```python
from build123d import *

# Parameters (mm, degrees)
F1_DEPTH = 40
F2_R     = 5
F3_W     = 50
F3_H     = 40
F4_DEPTH = 1


with BuildPart() as f1:
    # F0 (on Right) → F1 (new body, symmetric)
    with BuildSketch(Plane.YZ):
        with BuildLine():
            ThreePointArc((4.6023512578, 12.0836236967), (18.5654944992, 26.0467669382), (32.5286377407, 12.0836236967))
            Line((32.5286377407, 12.0836236967), (40.2273690835, 12.0836236967))
            Line((40.2273690835, 12.0836236967), (40.2273690835, 92.0836236967))
            Line((40.2273690835, 92.0836236967), (-29.7726309165, 92.0836236967))
            Line((-29.7726309165, 92.0836236967), (-39.7726309165, 42.0836236967))
            Line((-39.7726309165, 42.0836236967), (-79.7726309165, 42.0836236967))
            Line((-79.7726309165, 42.0836236967), (-79.7726309165, 12.0836236967))
            Line((-79.7726309165, 12.0836236967), (-68.3018244008, 12.0836236967))
            ThreePointArc((-68.3018244008, 12.0836236967), (-54.4831605593, 25.9022875381), (-40.6644967179, 12.0836236967))
            Line((-40.6644967179, 12.0836236967), (4.6023512578, 12.0836236967))
        make_face()
        with BuildLine():
            Line((-68.3018244008, 12.0836236967), (-40.6644967179, 12.0836236967))
            ThreePointArc((-40.6644967179, 12.0836236967), (-54.4831605593, 25.9022875381), (-68.3018244008, 12.0836236967))
        make_face()
        with BuildLine():
            ThreePointArc((-68.3018244008, 12.0836236967), (-54.4831605593, -1.7350401447), (-40.6644967179, 12.0836236967))
            Line((-40.6644967179, 12.0836236967), (-68.3018244008, 12.0836236967))
        make_face()
        with BuildLine():
            Line((4.6023512578, 12.0836236967), (32.5286377407, 12.0836236967))
            ThreePointArc((32.5286377407, 12.0836236967), (18.5654944992, 26.0467669382), (4.6023512578, 12.0836236967))
        make_face()
        with BuildLine():
            ThreePointArc((4.6023512578, 12.0836236967), (18.5654944992, -1.8795195447), (32.5286377407, 12.0836236967))
            Line((32.5286377407, 12.0836236967), (4.6023512578, 12.0836236967))
        make_face()
    extrude(amount=F1_DEPTH, both=True)

    # F2
    f2_edges = [f1.edges().sort_by_distance(p)[0] for p in [
        (-40, -34.772631, 67.083624),
        (0, -39.772631, 42.083624),
        (40, -34.772631, 67.083624),
        (0, -29.772631, 92.083624),
        (0, -79.772631, 42.083624),
        (-40, -79.772631, 27.083624),
        (0, -79.772631, 12.083624),
        (40, -79.772631, 27.083624),
        (0, -68.301824, 12.083624),
        (-40, -54.483161, -1.73504),
        (0, -40.664497, 12.083624),
        (40, -54.483161, -1.73504),
        (-40, -59.772631, 42.083624),
        (-40, -74.037228, 12.083624),
        (-40, -18.031073, 12.083624),
        (-40, 18.565494, -1.87952),
        (-40, 36.378003, 12.083624),
        (-40, 40.227369, 52.083624),
        (-40, 5.227369, 92.083624),
        (0, 40.227369, 92.083624),
        (40, 40.227369, 52.083624),
        (0, 40.227369, 12.083624),
        (40, -59.772631, 42.083624),
        (40, -74.037228, 12.083624),
        (40, -18.031073, 12.083624),
        (40, 18.565494, -1.87952),
        (40, 36.378003, 12.083624),
        (40, 5.227369, 92.083624),
    ]]
    fillet(f2_edges, radius=F2_R)

    # F3 (on face) → F4 (cut, symmetric)
    with BuildSketch(Plane.YZ.offset(40)):
        with Locations((3.8793236017, 61.9780325047)):
            Rectangle(F3_W, F3_H)
    extrude(amount=F4_DEPTH, both=True, mode=Mode.SUBTRACT)


solid = f1.part
```
Source: CAD feature listing. Evaluate the final solid. Frame: model axes, mm. A direction names the side the tool comes from. Give positions to 0.01 mm unless a question says otherwise; leave off trailing zeros. Order: outer loops, then holes, each group sorted by start corner. A loop starts at its lowest first (then second) coordinate and runs counter-clockwise, first axis right, second up. Notation, with made-up numbers: (35.5, 82) -> (88.5, 82) arc R26 cw to (88.5, 114) -> close; hole circle Ø8 at (19, 89). An arc over 180 degrees is marked (long way). Use a Markdown table: item, result.
Q1. Pull-direction query (Y, two-part tool) for faces 1 (the face through (38.496, -12.275, 13.509)), 2 (the face through (0.49, -34.714, 67.377)), 3 (the face through (38.496, -59.538, 40.658)); classes: +Y half, -Y half, draft (parallel to the pull), parting line (faces both ways), or undercut.
A:
| item | result |
|---|---|
| face 1 | undercut |
| face 2 | -Y half |
| face 3 | draft |
Q2. First-contact query: P1, Ø5, axis at x = 28.5, y = -43, coming from the +Z side; P2, Ø0.5, axis at x = 39.5, z = 61, coming from the +Y side; P3, Ø1.1, axis at x = 39.5, y = 1.5, coming from the +Z side. Flat tips, straight axial feed; report the tip coordinate or a pass-through.
A:
| item | result |
|---|---|
| P1 | z = 43.39 |
| P2 | y = 37.86 |
| P3 | z = 90.15 |
Q3. Access query for faces 4 (the face through (0, -16, 12.084)), 5 (the face through (38.496, -73.684, 13.509)), 6 (the face through (-38.496, -59.538, 40.658)). Directions: +Z, -Z, +X, -X, +Y, -Y. A direction counts if a zero-diameter tool reaches every point of the face in a straight line with its end or side. Return the directions, or none.
A:
| item | result |
|---|---|
| face 4 | -Z, +X, -X |
| face 5 | -Z, +X, -Y |
| face 6 | +Z, -X, -Y |
Q4. Section A-A (y = -22.5). Return the cut outline in (x, z), and give its area (3 significant figures).
A:
| item | result |
|---|---|
| outline | (-40, 17.08) arc R5 ccw to (-35, 12.08) -> (35, 12.08) arc R5 ccw to (40, 17.08) -> (40, 87.08) arc R5 ccw to (35, 92.08) -> (-35, 92.08) arc R5 ccw to (-40, 87.08) -> close |
| area | 6,380 mm^2 |
Q5. Section C-C (y = -7). Return the cut outline in (x, z).
A:
| item | result |
|---|---|
| outline | (-40, 17.08) arc R5 ccw to (-35, 12.08) -> (35, 12.08) arc R5 ccw to (40, 17.08) -> (40, 41.98) -> (39, 41.98) -> (39, 81.98) -> (40, 81.98) -> (40, 87.08) arc R5 ccw to (35, 92.08) -> (-35, 92.08) arc R5 ccw to (-40, 87.08) -> close |
Q6. Material intervals for line 1 (Z direction, x = -4, y = 4.5); line 2 (Y direction, x = 35.5, z = 8.5) (3 decimals); line 3 (Y direction, x = 21, z = 3), sorted ascending. Write a range as [from, to].
A:
| item | result |
|---|---|
| line 1 | [12.08, 92.08] |
| line 2 | [-67.804, -41.162], [5.096, 32.035] |
| line 3 | [-64.9, -44.07], [7.96, 29.17] |
Q7. Section B-B (x = 22). Return the cut outline in (y, z), and give its area (3 significant figures).
A:
| item | result |
|---|---|
| outline | (-79.77, 17.08) arc R5 ccw to (-74.77, 12.08) -> (-72.63, 12.08) arc R5 cw to (-67.81, 8.41) arc R13.82 ccw to (-41.16, 8.41) arc R5 cw to (-36.34, 12.08) -> (4.6, 12.08) arc R13.96 ccw to (32.53, 12.08) -> (35.23, 12.08) arc R5 ccw to (40.23, 17.08) -> (40.23, 87.08) arc R5 ccw to (35.23, 92.08) -> (-25.67, 92.08) arc R5 ccw to (-30.58, 88.06) -> (-38.97, 46.1) arc R5 cw to (-43.87, 42.08) -> (-74.77, 42.08) arc R5 ccw to (-79.77, 37.08) -> close |
| area | 7,940 mm^2 |
